Design review of the part built by this model. Coordinates are the model's own, in mm. Face numbers are marked on the shaded views. A direction names the side the tool comes from. Coordinates: 2 decimals unless noted, no trailing zeros. Order: outer loops, then holes, each group sorted by start corner. A loop starts at its lowest first (then second) coordinate and runs counter-clockwise, first axis right, second up. Notation, with made-up numbers: (46, -21) - (90, -21) arc R32 ccw to (90, 7) - close; hole circle Ø6 at (51.5, 86.5). An arc over 180 degrees is marked (long way). Write item = value, one per line. Start each with the question number.
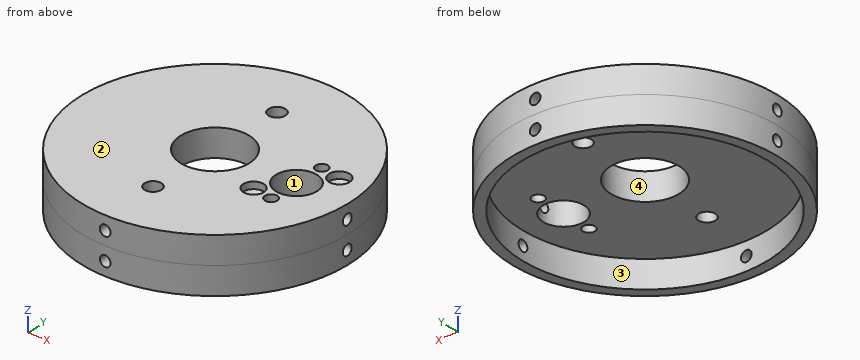
Autodesk Inventor part; units mm, degrees
ref_plane "Arbeitsebene1" through (-19.5, 0, 0) normal (1, 0, 0) x (0, 1, 0)
ref_plane "Arbeitsebene4" through (13.7886, 13.7886, 0) normal (0.7071, 0.7071, 0) x (-0.7071, 0.7071, 0)
ref_plane "XZ Plane" through (0, 0, 0) normal (0, 1, 0) x (-1, 0, 0)
sketch "Skizze1" plane through (0, 0, 0) normal (0, 0, 1) x (1, 0, 0)
  line L0 (-44.1689, 0) -> (40.5177, 0)
  line L1 (0, -38.9628) -> (0, 40.9677)
  circle A0 centre (0, 0) radius 19.5
  dimension "d0" = 39
extrude "Extrusion1" add sketch "Skizze1" along normal blind 4
hole "Bohrung1" at (0, 0, 4) direction (0, 0, -1) diameter 10 end through all
sketch "Skizze2" plane through (0, 0, 4) normal (0, 0, 1) x (1, 0, 0)
  circle A0 centre (0, 0) radius 5
  line L0 (-44.1689, 0) -> (40.5177, 0)
  line L1 (0, -38.9628) -> (0, 40.9677)
  point P0 (12, 0)
  dimension "d14" = 12
hole "Bohrung2" at (12, 0, 4) direction (0, 0, -1) diameter 6 end through all
sketch "Skizze5" plane through (0, 0, 4) normal (0, 0, 1) x (1, 0, 0)
  circle A0 centre (9, -4) radius 0.7
  circle A1 centre (15, 4) radius 0.7
hole "Bohrung4" at (9, -4, 4) at (15, 4, 4) direction (0, 0, -1) diameter 3 depth 1 tip angle 118
sketch "Skizze7" plane through (0, 0, 4) normal (0, 0, 1) x (1, 0, 0)
  line L0 (0, -38.9628) -> (0, 40.9677)
  line L1 (-44.1689, 0) -> (40.5177, 0)
  point P0 (12, -4.5)
  point P1 (12, 4.5)
  dimension "d39" = 12
  dimension "d40" = 9
hole "Bohrung5" at (12, -4.5, 4) at (12, 4.5, 4) direction (0, 0, -1) diameter 1.8 end through all
sketch "Skizze9" plane through (0, 0, 0) normal (0, 0, -1) x (-1, 0, 0)
  circle A0 centre (0, 0) radius 19.5
  circle A1 centre (0, 0) radius 18
  dimension "d58" = 1.5
extrude "Extrusion3" add sketch "Skizze9" along normal blind 4
ref_plane "Arbeitsebene1" through (-19.5, 0, 0) normal (1, 0, 0) x (0, 1, 0)
sketch "Skizze10" plane through (-19.5, 0, 0) normal (1, 0, 0) x (0, 1, 0)
  line L0 (-5.4, 4) -> (-3.6, 4)
  line L1 (3.6, 4) -> (5.4, 4)
  line L2 (-19.5, 4) -> (19.5, 4)
  line L3 (-3, 4) -> (3, 4)
  line L4 (-5, 4) -> (5, 4)
  line L5 (19.5, 4) -> (-19.5, 4)
  line L6 (-34.9563, 0) -> (28.576, 0)
  line L7 (0, -5.6) -> (0, 5.6)
  point P0 (0, 0)
  point P1 (-5.5, 4)
  point P2 (-2.5, 4)
  point P3 (2.5, 4)
  point P4 (5.5, 4)
  point P5 (0, 2)
  point P6 (0, -2)
  dimension "d63" = 2
  dimension "d104" = 4
hole "Bohrung7" at (-19.5, 0, 2) at (-19.5, 0, -2) direction (1, 0, 0) diameter 1.567 depth 6 tip angle 118
sketch "Skizze11" plane through (0, 0, 4) normal (0, 0, 1) x (1, 0, 0)
  circle A0 centre (12, -4.5) radius 0.9
  circle A1 centre (12, 4.5) radius 0.9
  circle A2 centre (9, -4) radius 1.5
  circle A3 centre (15, 4) radius 1.5
  circle A4 centre (12, 0) radius 3
  circle A5 centre (0, 0) radius 5
  circle A6 centre (0, 0) radius 19.5
  line L0 (0, 0) -> (-19.0596, 19.0596)
  line L1 (-27.3, 0) -> (27.3, 0)
  line L2 (0, -35.3992) -> (0, 31.2338)
  dimension "d71" = 45
ref_plane "Arbeitsebene4" through (13.7886, 13.7886, 0) normal (0.7071, 0.7071, 0) x (-0.7071, 0.7071, 0)
pattern_circular "Runde Anordnung1" count 4 over 360 about axis through (0, 0, 0) along (0, 0, 1) of "Bohrung7"
sketch "Skizze14" plane through (0, 0, 4) normal (0, 0, 1) x (1, 0, 0)
  line L0 (-27.3, 0) -> (27.3, 0)
  line L1 (0, -35.3992) -> (0, 31.2338)
  point P0 (0, 11)
  point P1 (0, -11)
  dimension "d96" = 22
hole "Bohrung10" at (0, 11, 4) at (0, -11, 4) direction (0, 0, -1) diameter 2.459 end through all
properties part number "13_1087_030"
Item 1: Add section C-C on x = -14.5. Give the boundary of the cut face in (y, z), plus the area to 3 significant figures.
Item 2: For the marked faces 3 and 4, list the 3-axis set-ups (+Z, -Z, +X, -X, +Y, -Y) from which the entire face can be reached by the end or side of a thin tool; tool diameter is ignored.
Item 3: For P1, Ø1.4, axis at y = 0, z = 2, coming from the +X side; P2, Ø4, axis at x = 9, y = -4, coming from the -Z side; P3, Ø1.1, axis at x = 12, y = -4.5, coming from the -Z side; P4, Ø1.8, axis at x = 0, z = 2, coming from the -Y side, all flat-tipped, find the tip position at first contact; note any pin that passes through.
Item 4: Add section A-A on z = -2. Give the boundary of the cut face in (x, y).
Item 5: Add section D-D on y = 11. Give the boundary of the cut face in (x, z).
Item 6: Mouldability with a two-part tool opening along Y and no side actions: class the marked faces 1 and 2 as +Y half, -Y half, draft (parallel to the pull), parting line (faces both ways), or undercut.
Item 7: For line 1 (Z direction, x = 0, y = -18.75); line 2 (Z direction, x = 8, y = -7); line 3 (Y direction, x = 11, z = 1.5), list the stretches that pass through material, from the lowest coordinate up.
Item 8: Add section B-B on y = -14. Give the boundary of the cut face in (x, z).
Worked out:
q1.outline = (-13.04, -4) - (-10.67, -4) - (-10.67, 0) - (10.67, 0) - (10.67, -4) - (13.04, -4) - (13.04, 4) - (-13.04, 4) - close; hole circle Ø1.57 at (0, 2)
q1.area = 121 mm2
q2.face_3 = -Z
q2.face_4 = +Z, -Z
q3.P1 = 9.08
q3.P2 = 0
q3.P3 = through
q3.P4 = -19.5
q4.outline = (-19.48, -0.78) arc R19.5 ccw to (-0.78, -19.48) - (-0.78, -17.98) arc R18 cw to (-17.98, -0.78) - close; (-19.48, 0.78) - (-17.98, 0.78) arc R18 cw to (-0.78, 17.98) - (-0.78, 19.48) arc R19.5 ccw to start; (0.78, -19.48) arc R19.5 ccw to (19.48, -0.78) - (17.98, -0.78) arc R18 cw to (0.78, -17.98) - close; (0.78, 17.98) arc R18 cw to (17.98, 0.78) - (19.48, 0.78) arc R19.5 ccw to (0.78, 19.48) - close
q5.outline = (-16.1, -4) - (-14.25, -4) - (-14.25, 0) - (-1.23, 0) - (-1.23, 4) - (-16.1, 4) - close; (1.23, 0) - (14.25, 0) - (14.25, -4) - (16.1, -4) - (16.1, 4) - (1.23, 4) - close
q6.face_1 = undercut
q6.face_2 = draft
q7.line_1 = -4 to -2.78, -1.22 to 1.22, 2.78 to 4
q7.line_2 = 0 to 4
q7.line_3 = -16.1 to -2.83, 2.83 to 16.1
q8.outline = (-13.57, -4) - (-11.31, -4) - (-11.31, 0) - (11.31, 0) - (11.31, -4) - (13.57, -4) - (13.57, 4) - (-13.57, 4) - close; hole circle Ø1.57 at (0, 2)
